Part print with two shaded views. Sizes in mm from the minimum x, y, z corner. A direction names the side the tool comes from. Give positions to 0.01 mm unless a question says otherwise; leave off trailing zeros. Order: outer loops, then holes, each group sorted by start corner. A loop starts at its lowest first (then second) coordinate and runs counter-clockwise, first axis right, second up. Notation, with made-up numbers: M 18,47.5 L 77,47.5 A26 ccw 77,67.5 Z; hole C -7.75,-37.5 d1. An arc over 180 degrees is marked long. Answer as CSV lines item,"result".
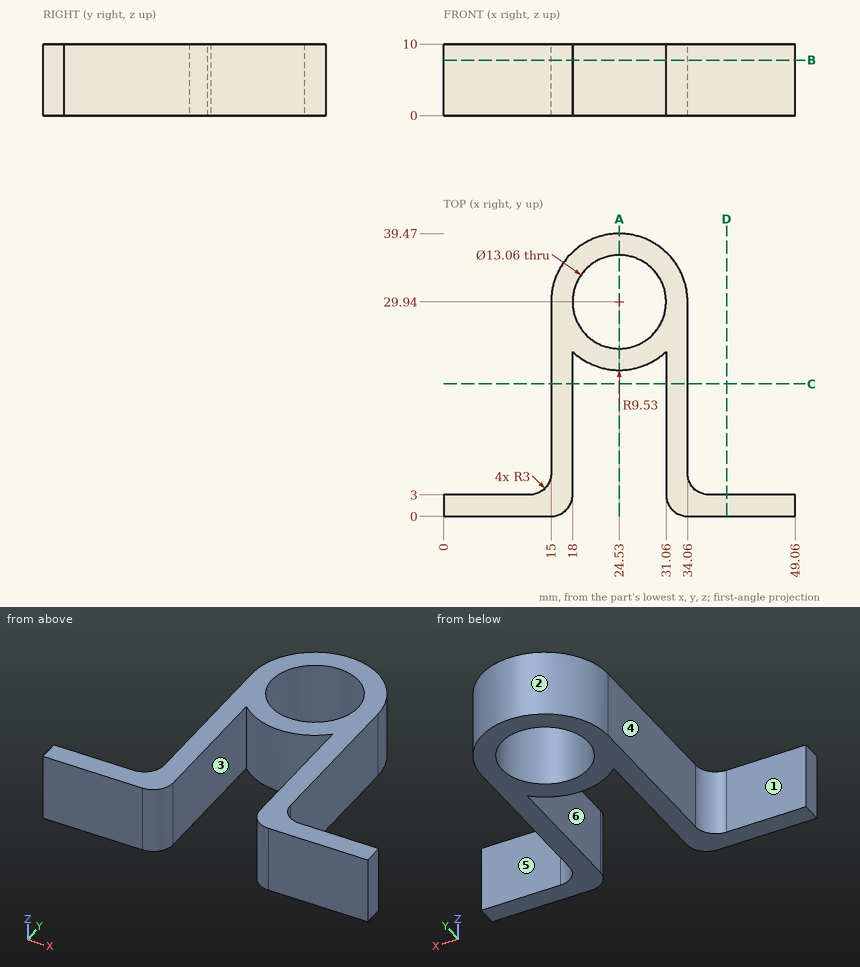
Item 1: Band-saw the part on B-B (z = 7.75). Give the cut face in (x, y).
Geometry says:
outline,"M 0,0 L 15,0 A3 ccw 18,3 L 18,23 A9.53 ccw 31.06,23 L 31.06,3 A3 ccw 34.06,0 L 49.06,0 L 49.06,3 L 37.06,3 A3 cw 34.06,6 L 34.06,29.94 A9.53 ccw 15,29.94 L 15,6 A3 cw 12,3 L 0,3 Z; hole C 24.53,29.94 d13.06"
Item 2: Band-saw the part on A-A (x = 24.53). Give the cut face in (y, z).
Geometry says:
outline,"M 20.41,0 L 23.41,0 L 23.41,10 L 20.41,10 Z; M 36.47,0 L 39.47,0 L 39.47,10 L 36.47,10 Z"
Item 3: Pull direction X, two halves, no side cores. Call the marked faces 1, 2 and 3: released by +X, released by -X, zero draft, split by the parting line, or undercut.
Geometry says:
face 1,"zero draft"
face 2,"split by the parting line"
face 3,"undercut"
Item 4: Probe line 1 along Y through (x, z) = (24.53, 7); line 2 along X through (y, z) = (14.5, 6); line 3 along X through (y, z) = (27.5, 0.5). List the from-to ranges inside material, lowest first. Write a range as from..to.
Geometry says:
line 1,"y = 20.41..23.41, 36.47..39.47"
line 2,"x = 15..18, 31.06..34.06"
line 3,"x = 15..18.47, 30.59..34.06"
Item 5: 3-axis set-ups, long thin cutter, end or side, ignore diameter. For the marked faces 4, 5 and 6: which of +Z, -Z, +X, -X, +Y, -Y reach the whole face in a straight line?
Geometry says:
face 4,"+Z, -Z, -X, +Y"
face 5,"+Z, -Z, +X, +Y"
face 6,"+Z, -Z, -Y"
Item 6: Band-saw the part on C-C (y = 18.5). Give the cut face in (x, z).
Geometry says:
outline,"M 15,0 L 18,0 L 18,10 L 15,10 Z; M 31.06,0 L 34.06,0 L 34.06,10 L 31.06,10 Z"
Item 7: Band-saw the part on D-D (x = 39.5). Give the cut face in (y, z), and give its area (3 significant figures).
Geometry says:
outline,"M 0,0 L 3,0 L 3,10 L 0,10 Z"
area,"30.0 mm2"
Item 8: Drop flat-ended pins along their axis: pin 1 (3 mm diameter, centred on y = 18, z = 4, fed in from -X); pin 2 (2 mm diameter, centred on y = 22, z = 3, fed in from +X); pin 3 (3 mm diameter, centred on x = 3, z = 6, fed in from +Y). Give the stop position or say it passes through.
Geometry says:
pin 1,"stops at x = 15"
pin 2,"stops at x = 34.06"
pin 3,"stops at y = 3"
